Work out the finished part from the listing and answer in its coordinate system (mm). Round coordinates to 2 decimals unless told otherwise and drop trailing zeros. Loops run counter-clockwise (first coordinate to the right, second up) from the corner with the lowest first, then second, coordinate; pieces in that order, holes last. Notation, with made-up numbers: (20, -21.75) - (74, -21.75) arc R14 cw to (74, 4.25) - close; hole circle Ø10 at (25, 14.5). An arc over 180 degrees is marked (long way). Use CSV: the item, a comma, the result in double quotes. Start each with the question number.
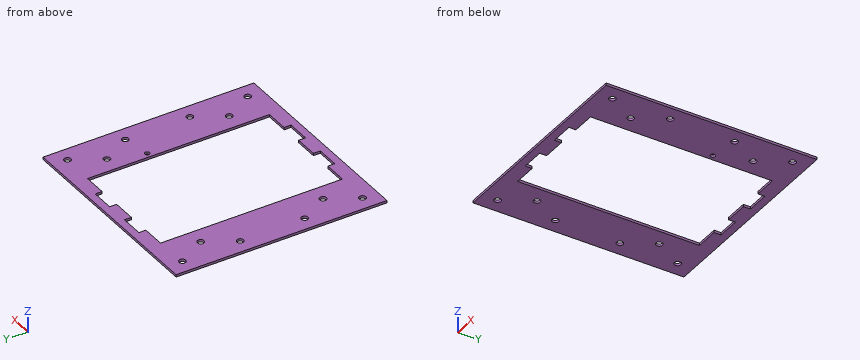
from build123d import *

# Parameters (mm, degrees)
SKETCH_1_W                      = 700
SKETCH_1_H                      = 700
CONNECTION_PLATE_DEPTH          = 8
SKETCH_2_W                      = 76
SKETCH_2_H                      = 300
ACCESS_WINDOW_DEPTH             = 990.981818015
SKETCH_3_W                      = 76
SKETCH_3_H                      = 300
CUT_EXTRUDE_2_DEPTH             = 990.981818015
SKETCH_4_W                      = 76
SKETCH_4_H                      = 300
CUT_EXTRUDE_3_DEPTH             = 990.981818015
SKETCH_5_W                      = 76
SKETCH_5_H                      = 300
CUT_EXTRUDE_4_DEPTH             = 990.981818015
SKETCH_6_R                      = 11
SHAFT_CLEARANCE_DEPTH           = 990.981818015
SKETCH_7_R                      = 11
CUT_EXTRUDE_6_DEPTH             = 990.981818015
SKETCH_8_R                      = 11
CUT_EXTRUDE_7_DEPTH             = 990.981818015
SKETCH_9_R                      = 11
CUT_EXTRUDE_8_DEPTH             = 990.981818015
SKETCH_10_R                     = 11
CUT_EXTRUDE_9_DEPTH             = 990.981818015
SKETCH_11_R                     = 11
CUT_EXTRUDE_10_DEPTH            = 990.981818015
SKETCH_12_R                     = 11
CUT_EXTRUDE_11_DEPTH            = 990.981818015
SKETCH_13_R                     = 11
CUT_EXTRUDE_12_DEPTH            = 990.981818015
SKETCH_14_R                     = 11
CUT_EXTRUDE_13_DEPTH            = 990.981818015
SKETCH_15_R                     = 11
CUT_EXTRUDE_14_DEPTH            = 990.981818015
SKETCH_16_R                     = 11
CUT_EXTRUDE_15_DEPTH            = 990.981818015
SKETCH_17_R                     = 11
CUT_EXTRUDE_16_DEPTH            = 990.981818015
SKETCH_18_W                     = 384
SKETCH_18_H                     = 604
FLOAT_INSTALLATION_WINDOW_DEPTH = 990.981818015
SKETCH_19_R                     = 8
COMMS_PASSAGE_DEPTH             = 990.981818015


with BuildPart() as part:
    # 草图1 → Connection_plate (new body)
    with BuildSketch(Plane.XY):
        with Locations((350, 350)):
            Rectangle(SKETCH_1_W, SKETCH_1_H)
    extrude(amount=CONNECTION_PLATE_DEPTH)

    # 草图2 → Access_window (cut, through all)
    with BuildSketch(Plane.XY.offset(8)):
        with Locations((273, 175)):
            Rectangle(SKETCH_2_W, SKETCH_2_H)
    extrude(amount=-ACCESS_WINDOW_DEPTH, mode=Mode.SUBTRACT)

    # 草图3 → 切除-拉伸2 (cut, through all)
    with BuildSketch(Plane.XY.offset(8)):
        with Locations((273, 525)):
            Rectangle(SKETCH_3_W, SKETCH_3_H)
    extrude(amount=-CUT_EXTRUDE_2_DEPTH, mode=Mode.SUBTRACT)

    # 草图4 → 切除-拉伸3 (cut, through all)
    with BuildSketch(Plane.XY.offset(8)):
        with Locations((427, 175)):
            Rectangle(SKETCH_4_W, SKETCH_4_H)
    extrude(amount=-CUT_EXTRUDE_3_DEPTH, mode=Mode.SUBTRACT)

    # 草图5 → 切除-拉伸4 (cut, through all)
    with BuildSketch(Plane.XY.offset(8)):
        with Locations((427, 525)):
            Rectangle(SKETCH_5_W, SKETCH_5_H)
    extrude(amount=-CUT_EXTRUDE_4_DEPTH, mode=Mode.SUBTRACT)

    # 草图6 → Shaft_clearance (cut, through all)
    with BuildSketch(Plane.XY.offset(8)):
        with Locations((48, 51)):
            Circle(SKETCH_6_R)
    extrude(amount=-SHAFT_CLEARANCE_DEPTH, mode=Mode.SUBTRACT)

    # 草图7 → 切除-拉伸6 (cut, through all)
    with BuildSketch(Plane.XY.offset(8)):
        with Locations((48, 243)):
            Circle(SKETCH_7_R)
    extrude(amount=-CUT_EXTRUDE_6_DEPTH, mode=Mode.SUBTRACT)

    # 草图8 → 切除-拉伸7 (cut, through all)
    with BuildSketch(Plane.XY.offset(8)):
        with Locations((48, 457)):
            Circle(SKETCH_8_R)
    extrude(amount=-CUT_EXTRUDE_7_DEPTH, mode=Mode.SUBTRACT)

    # 草图9 → 切除-拉伸8 (cut, through all)
    with BuildSketch(Plane.XY.offset(8)):
        with Locations((48, 649)):
            Circle(SKETCH_9_R)
    extrude(amount=-CUT_EXTRUDE_8_DEPTH, mode=Mode.SUBTRACT)

    # 草图10 → 切除-拉伸9 (cut, through all)
    with BuildSketch(Plane.XY.offset(8)):
        with Locations((103.43, 147)):
            Circle(SKETCH_10_R)
    extrude(amount=-CUT_EXTRUDE_9_DEPTH, mode=Mode.SUBTRACT)

    # 草图11 → 切除-拉伸10 (cut, through all)
    with BuildSketch(Plane.XY.offset(8)):
        with Locations((103.43, 553)):
            Circle(SKETCH_11_R)
    extrude(amount=-CUT_EXTRUDE_10_DEPTH, mode=Mode.SUBTRACT)

    # 草图12 → 切除-拉伸11 (cut, through all)
    with BuildSketch(Plane.XY.offset(8)):
        with Locations((652, 51)):
            Circle(SKETCH_12_R)
    extrude(amount=-CUT_EXTRUDE_11_DEPTH, mode=Mode.SUBTRACT)

    # 草图13 → 切除-拉伸12 (cut, through all)
    with BuildSketch(Plane.XY.offset(8)):
        with Locations((652, 243)):
            Circle(SKETCH_13_R)
    extrude(amount=-CUT_EXTRUDE_12_DEPTH, mode=Mode.SUBTRACT)

    # 草图14 → 切除-拉伸13 (cut, through all)
    with BuildSketch(Plane.XY.offset(8)):
        with Locations((652, 457)):
            Circle(SKETCH_14_R)
    extrude(amount=-CUT_EXTRUDE_13_DEPTH, mode=Mode.SUBTRACT)

    # 草图15 → 切除-拉伸14 (cut, through all)
    with BuildSketch(Plane.XY.offset(8)):
        with Locations((652, 649)):
            Circle(SKETCH_15_R)
    extrude(amount=-CUT_EXTRUDE_14_DEPTH, mode=Mode.SUBTRACT)

    # 草图16 → 切除-拉伸15 (cut, through all)
    with BuildSketch(Plane.XY.offset(8)):
        with Locations((596.57, 147)):
            Circle(SKETCH_16_R)
    extrude(amount=-CUT_EXTRUDE_15_DEPTH, mode=Mode.SUBTRACT)

    # 草图17 → 切除-拉伸16 (cut, through all)
    with BuildSketch(Plane.XY.offset(8)):
        with Locations((596.57, 553)):
            Circle(SKETCH_17_R)
    extrude(amount=-CUT_EXTRUDE_16_DEPTH, mode=Mode.SUBTRACT)

    # 草图18 → Float_installation_window (cut, through all)
    with BuildSketch(Plane.XY.offset(8)):
        with Locations((350, 350)):
            Rectangle(SKETCH_18_W, SKETCH_18_H)
    extrude(amount=-FLOAT_INSTALLATION_WINDOW_DEPTH, mode=Mode.SUBTRACT)

    # 草图19 → Comms_passage (cut, through all)
    with BuildSketch(Plane.XY.offset(8)):
        with Locations((560, 442.45)):
            Circle(SKETCH_19_R)
    extrude(amount=-COMMS_PASSAGE_DEPTH, mode=Mode.SUBTRACT)


solid = part.part
Item 1: Find the intervals of material crossed by probe 1 along Y at (x, z) = (652, 2.5); probe 2 along X at (y, z) = (375.5, 4.5); probe 3 along X at (y, z) = (649, 2.75), in increasing order. Write a range as [from, to].
Item 2: A cutting plane is placed at A-A (x = 483). Determine the outline of the cut face in (y, z).
Item 3: A cutting plane is placed at D-D (y = 593). Determine the outline of the cut face in (x, z).
Item 4: A cutting plane is placed at C-C (x = 48). Determine the outline of the cut face in (y, z), plus the area to 3 significant figures.
Item 5: A cutting plane is placed at B-B (y = 147). Determine the outline of the cut face in (x, z).
Result sheet:
1,probe 1,"[0, 40], [62, 232], [254, 446], [468, 638], [660, 700]"
1,probe 2,"[0, 158], [542, 700]"
1,probe 3,"[0, 37], [59, 158], [542, 641], [663, 700]"
2,outline,"(0, 0) - (48, 0) - (48, 8) - (0, 8) - close; (652, 0) - (700, 0) - (700, 8) - (652, 8) - close"
3,outline,"(0, 0) - (158, 0) - (158, 8) - (0, 8) - close; (542, 0) - (700, 0) - (700, 8) - (542, 8) - close"
4,outline,"(0, 0) - (40, 0) - (40, 8) - (0, 8) - close; (62, 0) - (232, 0) - (232, 8) - (62, 8) - close; (254, 0) - (446, 0) - (446, 8) - (254, 8) - close; (468, 0) - (638, 0) - (638, 8) - (468, 8) - close; (660, 0) - (700, 0) - (700, 8) - (660, 8) - close"
4,area,"4,900 mm^2"
5,outline,"(0, 0) - (92.43, 0) - (92.43, 8) - (0, 8) - close; (114.43, 0) - (158, 0) - (158, 8) - (114.43, 8) - close; (542, 0) - (585.57, 0) - (585.57, 8) - (542, 8) - close; (607.57, 0) - (700, 0) - (700, 8) - (607.57, 8) - close"
